```python
from build123d import *

# Parameters (mm, degrees)
BOSS_EXTRUDE1_DEPTH          = 2
BOSS_EXTRUDE1_2_DEPTH        = 2
BASE_W                       = 20
BASE_H                       = 70
BOSS_EXTRUDE2_DEPTH          = 2
F_3_CM_HANG_LOWER_W          = 50
F_3_CM_HANG_LOWER_H          = 30
BOSS_EXTRUDE3_DEPTH          = 2
F_3CM_HANG_UPPER_W           = 45
F_3CM_HANG_UPPER_H           = 30
BOSS_EXTRUDE4_DEPTH          = 2
LOWER_HOLDER_2ND_EXTEND_W    = 40
LOWER_HOLDER_2ND_EXTEND_H    = 5
BOSS_EXTRUDE5_DEPTH          = 2
UPPER_HOLDER_2ND_EXTEND_W    = 45
UPPER_HOLDER_2ND_EXTEND_H    = 5
BOSS_EXTRUDE6_DEPTH          = 2
FLATTEN_BENDS1_START         = -10
FLATTEN_BENDS1_DEPTH         = 50
FLATTEN_BENDS1_START_2       = -8.5
FLATTEN_BENDS1_2_OUTLINE_W   = 3.7366
FLATTEN_BENDS1_2_OUTLINE_H   = 2
FLATTEN_BENDS1_2_DEPTH       = 1
FLATTEN_BENDS1_START_3       = 37.5
FLATTEN_BENDS1_3_OUTLINE_W   = 3.7366
FLATTEN_BENDS1_3_OUTLINE_H   = 2
FLATTEN_BENDS1_3_DEPTH       = 1
FLATTEN_BENDS1_START_4       = -7.5
FLATTEN_BENDS1_4_OUTLINE_W   = 33.509289802
FLATTEN_BENDS1_4_OUTLINE_H   = 2
FLATTEN_BENDS1_4_OUTLINE_W_2 = 24.5268
FLATTEN_BENDS1_4_DEPTH       = 45
FLATTEN_BENDS1_5_OUTLINE_W   = 32.518044901
FLATTEN_BENDS1_5_OUTLINE_H   = 2
FLATTEN_BENDS1_5_DEPTH       = 39.999999999
FLATTEN_BENDS1_START_5       = 11
FLATTEN_BENDS1_6_OUTLINE_W   = 26.2634
FLATTEN_BENDS1_6_OUTLINE_H   = 2
FLATTEN_BENDS1_6_DEPTH       = 29
FLATTEN_BENDS1_START_6       = 31
FLATTEN_BENDS1_7_OUTLINE_W   = 3.7366
FLATTEN_BENDS1_7_OUTLINE_H   = 2
FLATTEN_BENDS1_7_DEPTH       = 9
FLATTEN_BENDS1_8_OUTLINE_W   = 0.991244901
FLATTEN_BENDS1_8_OUTLINE_H   = 2
FLATTEN_BENDS1_8_DEPTH       = 20
PROCESS_BENDS1_START         = -7.5
PROCESS_BENDS1_DEPTH         = 45
PROCESS_BENDS1_START_2       = -10
PROCESS_BENDS1_2_DEPTH       = 50
PROCESS_BENDS1_START_3       = 11
PROCESS_BENDS1_3_DEPTH       = 29
PROCESS_BENDS1_4_OUTLINE_W   = 2
PROCESS_BENDS1_4_OUTLINE_H   = 24.5268
PROCESS_BENDS1_4_DEPTH       = 45
PROCESS_BENDS1_5_DEPTH       = 39.999999999
PROCESS_BENDS1_6_OUTLINE_W   = 2
PROCESS_BENDS1_6_OUTLINE_H   = 26.2634
PROCESS_BENDS1_6_DEPTH       = 29
PROCESS_BENDS1_7_DEPTH       = 20
PROCESS_BENDS1_START_4       = 31
PROCESS_BENDS1_8_OUTLINE_W   = 2
PROCESS_BENDS1_8_OUTLINE_H   = 3.7366
PROCESS_BENDS1_8_DEPTH       = 9


# Read off the part's stored shape, not the designer's step: Flatten-Bends1, Process-Bends1
with BuildPart() as part:
    # hook → Boss-Extrude1 (new body)
    with BuildSketch(Plane.XY):
        with BuildLine():
            Line((-10, 35), (-10, 25))
            Line((-10, 25), (-58.535533906, 73.535533906))
            ThreePointArc((-58.535533906, 73.535533906), (-59.619397663, 75.15765065), (-60, 77.071067812))
            Line((-60, 77.071067812), (-60, 85))
            ThreePointArc((-60, 85), (-58.535533906, 88.535533906), (-55, 90))
            Line((-55, 90), (-27.5, 90))
            ThreePointArc((-27.5, 90), (-25.732233047, 89.267766953), (-25, 87.5))
            Line((-25, 87.5), (-24.999999999, 76.499999999))
            ThreePointArc((-24.999999999, 76.499999999), (-25.439339828, 75.439339828), (-26.499999999, 74.999999999))
            Line((-26.499999999, 74.999999999), (-28.499999999, 74.999999999))
            ThreePointArc((-28.499999999, 74.999999999), (-29.560660171, 75.439339828), (-29.999999999, 76.499999999))
            Line((-29.999999999, 76.499999999), (-29.999999999, 84.999999999))
            Line((-29.999999999, 84.999999999), (-49.999999999, 84.999999999))
            Line((-49.999999999, 84.999999999), (-50, 77.071067812))
            ThreePointArc((-50, 77.071067812), (-49.619397663, 75.15765065), (-48.535533906, 73.535533906))
            Line((-48.535533906, 73.535533906), (-10, 35))
        make_face()
    extrude(amount=-BOSS_EXTRUDE1_DEPTH)



with BuildPart() as body_2:
    # hook → Boss-Extrude1 2 (new body)
    with BuildSketch(Plane.XY):
        with BuildLine():
            Line((48.535533906, 73.535533906), (40, 65))
            Line((40, 65), (40, 35))
            Line((40, 35), (10, 35))
            Line((10, 35), (10, 25))
            Line((10, 25), (47.5, 25))
            ThreePointArc((47.5, 25), (49.267766953, 25.732233047), (50, 27.5))
            Line((50, 27.5), (50, 65))
            Line((50, 65), (58.535533906, 73.535533906))
            ThreePointArc((58.535533906, 73.535533906), (59.619397663, 75.15765065), (60, 77.071067812))
            Line((60, 77.071067812), (60, 85))
            ThreePointArc((60, 85), (58.535533906, 88.535533906), (55, 90))
            Line((55, 90), (27.5, 90))
            ThreePointArc((27.5, 90), (25.732233047, 89.267766953), (25, 87.5))
            Line((25, 87.5), (24.999999999, 76.499999999))
            ThreePointArc((24.999999999, 76.499999999), (25.439339828, 75.439339828), (26.499999999, 74.999999999))
            Line((26.499999999, 74.999999999), (28.499999999, 74.999999999))
            ThreePointArc((28.499999999, 74.999999999), (29.560660171, 75.439339828), (29.999999999, 76.499999999))
            Line((29.999999999, 76.499999999), (29.999999999, 84.999999999))
            Line((29.999999999, 84.999999999), (49.999999999, 84.999999999))
            Line((49.999999999, 84.999999999), (50, 77.071067812))
            ThreePointArc((50, 77.071067812), (49.619397663, 75.15765065), (48.535533906, 73.535533906))
        make_face()
    extrude(amount=-BOSS_EXTRUDE1_2_DEPTH)


with BuildPart() as part_1:
    add(part.part)

    add(body_2.part)  # Boss-Extrude2 merges body 2
    # base → Boss-Extrude2 (add)
    with BuildSketch(Plane.XY):
        Rectangle(BASE_W, BASE_H)
    extrude(amount=-BOSS_EXTRUDE2_DEPTH)

    # 3cm hang upper → Boss-Extrude4 (add)
    with BuildSketch(Plane(origin=(0, 35, 0), x_dir=(1, 0, 0), z_dir=(0, 1, 0))):
        with Locations((15, -15)):
            Rectangle(F_3CM_HANG_UPPER_W, F_3CM_HANG_UPPER_H)
    extrude(amount=-BOSS_EXTRUDE4_DEPTH)


with BuildPart() as body_2_2:
    # 3 cm hang lower → Boss-Extrude3 (new body)
    with BuildSketch(Plane(origin=(0, -35, 0), x_dir=(1, 0, 0), z_dir=(0, 1, 0))):
        with Locations((15, -15)):
            Rectangle(F_3_CM_HANG_LOWER_W, F_3_CM_HANG_LOWER_H)
    extrude(amount=BOSS_EXTRUDE3_DEPTH)


    add(part_1.part)  # Boss-Extrude5 merges part
    # lower holder 2nd extend → Boss-Extrude5 (add)
    with BuildSketch(Plane.XY.offset(30)):
        with Locations((10, -30.5)):
            Rectangle(LOWER_HOLDER_2ND_EXTEND_W, LOWER_HOLDER_2ND_EXTEND_H)
    extrude(amount=-BOSS_EXTRUDE5_DEPTH)

    # upper holder 2nd extend → Boss-Extrude6 (add)
    with BuildSketch(Plane.XY.offset(30)):
        with Locations((15, 30.5)):
            Rectangle(UPPER_HOLDER_2ND_EXTEND_W, UPPER_HOLDER_2ND_EXTEND_H)
    extrude(amount=-BOSS_EXTRUDE6_DEPTH)

    # Flatten-Bends1 outline → Flatten-Bends1 (cut)
    with BuildSketch(Plane.YZ.offset(FLATTEN_BENDS1_START)):
        Polygon((-33, 0), (-33, 28), (-28, 28), (-28, 30), (-35, 30), (-35, 0), align=None)
        Polygon((33, 28), (33, 0), (35, 0), (35, 30), (28, 30), (28, 28), align=None)
    extrude(amount=FLATTEN_BENDS1_DEPTH, mode=Mode.SUBTRACT)

    # Flatten-Bends1 2 outline → Flatten-Bends1 2 (cut)
    with BuildSketch(Plane.YZ.offset(FLATTEN_BENDS1_START_2)):
        with Locations((33.1317, -1)):
            Rectangle(FLATTEN_BENDS1_2_OUTLINE_W, FLATTEN_BENDS1_2_OUTLINE_H)
    extrude(amount=FLATTEN_BENDS1_2_DEPTH, mode=Mode.SUBTRACT)

    # Flatten-Bends1 3 outline → Flatten-Bends1 3 (cut)
    with BuildSketch(Plane.YZ.offset(FLATTEN_BENDS1_START_3)):
        with Locations((33.1317, -1)):
            Rectangle(FLATTEN_BENDS1_3_OUTLINE_W, FLATTEN_BENDS1_3_OUTLINE_H)
    extrude(amount=FLATTEN_BENDS1_3_DEPTH, mode=Mode.SUBTRACT)

    # Flatten-Bends1 4 outline → Flatten-Bends1 4 (add)
    with BuildSketch(Plane.YZ.offset(FLATTEN_BENDS1_START_4)):
        with Locations((51.754644901, -1)):
            Rectangle(FLATTEN_BENDS1_4_OUTLINE_W, FLATTEN_BENDS1_4_OUTLINE_H)
        with Locations((-48.254644901, -1)):
            Rectangle(FLATTEN_BENDS1_4_OUTLINE_W_2, FLATTEN_BENDS1_4_OUTLINE_H)
    extrude(amount=FLATTEN_BENDS1_4_DEPTH)

    # Flatten-Bends1 5 outline → Flatten-Bends1 5 (add)
    with BuildSketch(Plane.YZ.offset(FLATTEN_BENDS1_START)):
        with Locations((-52.250267351, -1)):
            Rectangle(FLATTEN_BENDS1_5_OUTLINE_W, FLATTEN_BENDS1_5_OUTLINE_H)
    extrude(amount=FLATTEN_BENDS1_5_DEPTH)

    # Flatten-Bends1 6 outline → Flatten-Bends1 6 (add)
    with BuildSketch(Plane.YZ.offset(FLATTEN_BENDS1_START_5)):
        with Locations((-47.386344901, -1)):
            Rectangle(FLATTEN_BENDS1_6_OUTLINE_W, FLATTEN_BENDS1_6_OUTLINE_H)
    extrude(amount=FLATTEN_BENDS1_6_DEPTH)

    # Flatten-Bends1 7 outline → Flatten-Bends1 7 (add)
    with BuildSketch(Plane.YZ.offset(FLATTEN_BENDS1_START_6)):
        with Locations((-62.386344901, -1)):
            Rectangle(FLATTEN_BENDS1_7_OUTLINE_W, FLATTEN_BENDS1_7_OUTLINE_H)
    extrude(amount=FLATTEN_BENDS1_7_DEPTH)

    # Flatten-Bends1 8 outline → Flatten-Bends1 8 (add)
    with BuildSketch(Plane.YZ.offset(FLATTEN_BENDS1_START)):
        with Locations((-35.495622451, -1)):
            Rectangle(FLATTEN_BENDS1_8_OUTLINE_W, FLATTEN_BENDS1_8_OUTLINE_H)
    extrude(amount=FLATTEN_BENDS1_8_DEPTH)

    # Process-Bends1 outline → Process-Bends1 (cut)
    with BuildSketch(Plane.YZ.offset(PROCESS_BENDS1_START)):
        with BuildLine():
            Line((68.509289802, 0), (34.899002398, 0))
            ThreePointArc((34.899002398, 0), (33.917667209, -1.443395312), (32.2634, -2))
            Line((32.2634, -2), (68.509289802, -2))
            Line((68.509289802, -2), (68.509289802, 0))
        make_face()
        with BuildLine():
            Line((-68.509289802, 0), (-68.509289802, -2))
            Line((-68.509289802, -2), (-32.2634, -2))
            ThreePointArc((-32.2634, -2), (-33.917667209, -1.443395312), (-34.899002398, 0))
            Line((-34.899002398, 0), (-68.509289802, 0))
        make_face()
    extrude(amount=PROCESS_BENDS1_DEPTH, mode=Mode.SUBTRACT)

    # Process-Bends1 2 outline → Process-Bends1 2 (cut)
    with BuildSketch(Plane.YZ.offset(PROCESS_BENDS1_START_2)):
        with BuildLine():
            Line((-68.509289802, 0), (-68.509289802, -2))
            Line((-68.509289802, -2), (-32.2634, -2))
            ThreePointArc((-32.2634, -2), (-33.917667209, -1.443395312), (-34.899002398, 0))
            Line((-34.899002398, 0), (-68.509289802, 0))
        make_face()
    extrude(amount=PROCESS_BENDS1_2_DEPTH, mode=Mode.SUBTRACT)

    # Process-Bends1 3 outline → Process-Bends1 3 (cut)
    with BuildSketch(Plane.YZ.offset(PROCESS_BENDS1_START_3)):
        with BuildLine():
            Line((-34.254644901, 0), (-34.899002398, 0))
            ThreePointArc((-34.899002398, 0), (-34.646082873, -0.609431903), (-34.254644901, -1.140611576))
            Line((-34.254644901, -1.140611576), (-34.254644901, 0))
        make_face()
    extrude(amount=PROCESS_BENDS1_3_DEPTH, mode=Mode.SUBTRACT)

    # Process-Bends1 4 outline → Process-Bends1 4 (add)
    with BuildSketch(Plane.YZ.offset(PROCESS_BENDS1_START)):
        with BuildLine():
            Line((32.2634, 30), (28, 30))
            Line((28, 30), (28, 28))
            Line((28, 28), (32.2634, 28))
            ThreePointArc((32.2634, 28), (32.784254855, 27.784254855), (33, 27.2634))
            Line((33, 27.2634), (33, 0.7366))
            ThreePointArc((33, 0.7366), (32.784254855, 0.215745145), (32.2634, 0))
            Line((32.2634, 0), (34.899002398, 0))
            ThreePointArc((34.899002398, 0), (34.974633029, 0.364854094), (35, 0.7366))
            Line((35, 0.7366), (35, 27.2634))
            ThreePointArc((35, 27.2634), (34.198468417, 29.198468417), (32.2634, 30))
        make_face()
        with Locations((-34, 14)):
            Rectangle(PROCESS_BENDS1_4_OUTLINE_W, PROCESS_BENDS1_4_OUTLINE_H)
    extrude(amount=PROCESS_BENDS1_4_DEPTH)

    # Process-Bends1 5 outline → Process-Bends1 5 (add)
    with BuildSketch(Plane.YZ.offset(PROCESS_BENDS1_START_2)):
        with BuildLine():
            Line((-28, 30), (-32.2634, 30))
            ThreePointArc((-32.2634, 30), (-34.198468417, 29.198468417), (-35, 27.2634))
            Line((-35, 27.2634), (-35, 1.7366))
            Line((-35, 1.7366), (-33, 1.7366))
            Line((-33, 1.7366), (-33, 27.2634))
            ThreePointArc((-33, 27.2634), (-32.784254855, 27.784254855), (-32.2634, 28))
            Line((-32.2634, 28), (-28, 28))
            Line((-28, 28), (-28, 30))
        make_face()
    extrude(amount=PROCESS_BENDS1_5_DEPTH)

    # Process-Bends1 6 outline → Process-Bends1 6 (add)
    with BuildSketch(Plane.YZ.offset(PROCESS_BENDS1_START_3)):
        with Locations((-34, 13.1317)):
            Rectangle(PROCESS_BENDS1_6_OUTLINE_W, PROCESS_BENDS1_6_OUTLINE_H)
    extrude(amount=PROCESS_BENDS1_6_DEPTH)

    # Process-Bends1 7 outline → Process-Bends1 7 (add)
    with BuildSketch(Plane.YZ.offset(PROCESS_BENDS1_START_2)):
        with BuildLine():
            Line((-33, 0.7366), (-33, 1.7366))
            Line((-33, 1.7366), (-35, 1.7366))
            Line((-35, 1.7366), (-35, 0.7366))
            ThreePointArc((-35, 0.7366), (-34.974633029, 0.364854094), (-34.899002398, 0))
            Line((-34.899002398, 0), (-32.2634, 0))
            ThreePointArc((-32.2634, 0), (-32.784254855, 0.215745145), (-33, 0.7366))
        make_face()
    extrude(amount=PROCESS_BENDS1_7_DEPTH)

    # Process-Bends1 8 outline → Process-Bends1 8 (add)
    with BuildSketch(Plane.YZ.offset(PROCESS_BENDS1_START_4)):
        with Locations((-34, 28.1317)):
            Rectangle(PROCESS_BENDS1_8_OUTLINE_W, PROCESS_BENDS1_8_OUTLINE_H)
    extrude(amount=PROCESS_BENDS1_8_DEPTH)


solid = body_2_2.part
```
Input: part model. Units: mm. Frame: model coordinates. A direction names the side the tool comes from. Give positions to 0.01 mm unless a question says otherwise; leave off trailing zeros. Order: outer loops, then holes, each group sorted by start corner. A loop starts at its lowest first (then second) coordinate and runs counter-clockwise, first axis right, second up. Notation, with made-up numbers: M 58.5,25.5 L 69.5,25.5 A20 ccw 69.5,64.5 Z; hole C 53,-19.5 d2. An arc over 180 degrees is marked long. Return JSON: item names as keys, results as strings.
Item 1: Cut plane D-D (y = 7). Return loops of the section in (x, z), then the cut area to 3 significant figures.
Solutions:
{"outline": "M -10,-2 L 10,-2 L 10,0 L -10,0 Z", "area": "40.0 mm^2"}
Item 2: Ray query, probe 1 along Y at (x, z) = (23.5, 5.5); probe 2 along Z at (x, y) = (51.5, 72.5); probe 3 along X at (y, z) = (52, -1). Return the intervals inside material, ascending.
Solutions:
{"probe 1": "-35 to -33, 33 to 35", "probe 2": "-2 to 0", "probe 3": "-37 to -27, 40 to 50"}
Item 3: Access query for faces 1 (the flat face through (15, 30, 28)), 2 (the flat face through (44, 69, -1)), 3 (the flat face through (-10, -14, -1)), 4 (the cylindrical face through (9.72, -34.177, 29.22)). Directions: +Z, -Z, +X, -X, +Y, -Y. A direction counts if a zero-diameter tool reaches every point of the face in a straight line with its end or side. Return the directions, or none.
Solutions:
{"face 1": "+X, -X", "face 2": "+Z, -Z", "face 3": "+Z, -Z, -X, -Y", "face 4": "+Z, -X, -Y"}
Item 4: Cut plane C-C (x = -20). Return loops of the section in (y, z), then the cut area to 3 significant figures.
Solutions:
{"outline": "M 35,-2 L 45,-2 L 45,0 L 35,0 Z", "area": "20.0 mm^2"}
Item 5: Cut plane A-A (y = 56). Return loops of the section in (x, z).
Solutions:
{"outline": "M -41,-2 L -31,-2 L -31,0 L -41,0 Z; M 40,-2 L 50,-2 L 50,0 L 40,0 Z"}
Item 6: First-contact query: P1, Ø1.1, axis at y = -20, z = 0.5, coming from the +X side; P2, Ø7.5, axis at y = 33, z = 21, coming from the +X side; P3, Ø10, axis at x = -28.5, y = 59, coming from the +Z side. Flat tips, straight axial feed; report the tip coordinate or a pass-through.
Solutions:
{"P1": "x = 10", "P2": "x = 37.5", "P3": "z = 0"}
Item 7: Pull-direction query (Y, two-part tool) for faces 5 (the flat face through (15, 35, 14)), 6 (the flat face through (-34, 49, -1)), 7 (the flat face through (10, -30, 28)); classes: +Y half, -Y half, draft (parallel to the pull), parting line (faces both ways), or undercut.
Solutions:
{"face 5": "+Y half", "face 6": "-Y half", "face 7": "undercut"}
Item 8: Cut plane B-B (z = 10). Return loops of the section in (x, y).
Solutions:
{"outline": "M -10,-35 L 40,-35 L 40,-33 L -10,-33 Z; M -7.5,33 L 37.5,33 L 37.5,35 L -7.5,35 Z"}
